Source: three-view drawing plus pictorial views. Frame: mm from the lowest corner of the part. Coordinates: 2 decimals unless noted, no trailing zeros. Loops run counter-clockwise (first coordinate to the right, second up) from the corner with the lowest first, then second, coordinate; pieces in that order, holes last. Notation, with made-up numbers: (75.25, 36) - (114.25, 36) arc R21 ccw to (114.25, 46) - close; hole circle Ø5 at (2, 70.5). An arc over 180 degrees is marked (long way). Return JSON: item names as keys, results as strings.
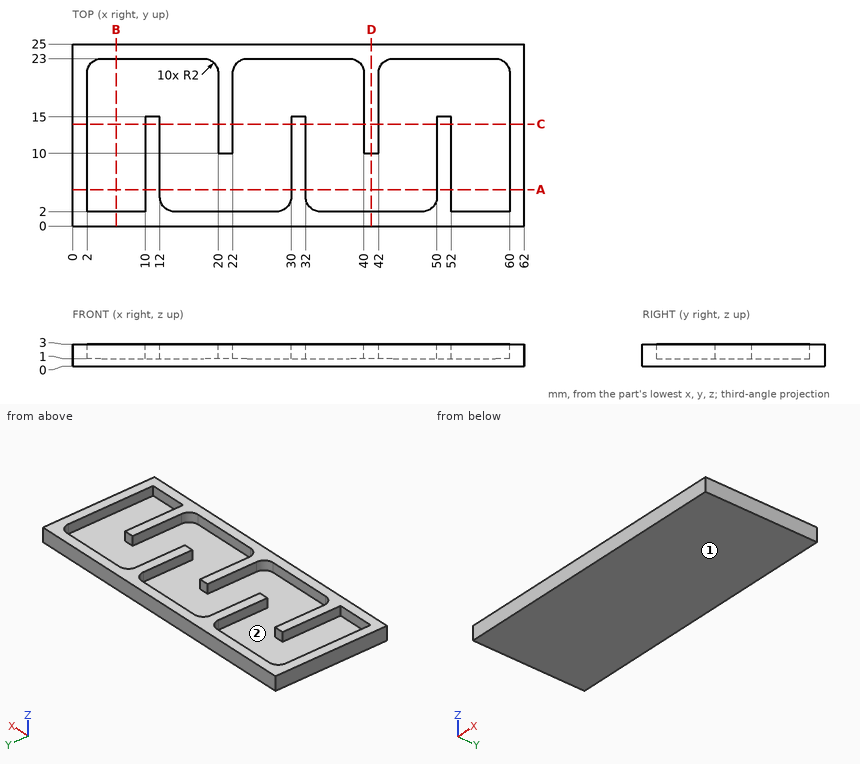
Item 1: Mould query, pull axis X, two halves, no side actions, for the marked faces 1 and 2. Classes: +X half, -X half, draft (parallel to the pull), parting line (faces both ways), or undercut.
Worked out:
{"face 1": "draft", "face 2": "undercut"}
Item 2: First-contact query: pin 1 Ø5 at (x, y) = (15, 20) entering from +Z. Flat tip, straight axial feed; report the tip coordinate or a pass-through.
Worked out:
{"pin 1": "z = 1"}
Item 3: Section query C-C, the plane y = 14. Return loops of the section in (x, z).
Worked out:
{"outline": "(0, 0) - (62, 0) - (62, 3) - (60, 3) - (60, 1) - (52, 1) - (52, 3) - (50, 3) - (50, 1) - (42, 1) - (42, 3) - (40, 3) - (40, 1) - (32, 1) - (32, 3) - (30, 3) - (30, 1) - (22, 1) - (22, 3) - (20, 3) - (20, 1) - (12, 1) - (12, 3) - (10, 3) - (10, 1) - (2, 1) - (2, 3) - (0, 3) - close"}
Item 4: Ray query, probe 1 along X at (y, z) = (9, 1.8); probe 2 along X at (y, z) = (16, 1.3); probe 3 along Y at (x, z) = (44, 1.25). Return the intervals inside material, ascending. Write a range as from..to.
Worked out:
{"probe 1": "0..2, 10..12, 30..32, 50..52, 60..62", "probe 2": "0..2, 20..22, 40..42, 60..62", "probe 3": "0..2, 23..25"}
Item 5: Section query A-A, the plane y = 5. Return loops of the section in (x, z).
Worked out:
{"outline": "(0, 0) - (62, 0) - (62, 3) - (60, 3) - (60, 1) - (52, 1) - (52, 3) - (50, 3) - (50, 1) - (32, 1) - (32, 3) - (30, 3) - (30, 1) - (12, 1) - (12, 3) - (10, 3) - (10, 1) - (2, 1) - (2, 3) - (0, 3) - close"}
Item 6: Section query D-D, the plane x = 41. Return loops of the section in (y, z), and give its area (3 significant figures).
Worked out:
{"outline": "(0, 0) - (25, 0) - (25, 3) - (10, 3) - (10, 1) - (2, 1) - (2, 3) - (0, 3) - close", "area": "59.0 mm^2"}
Item 7: Section query B-B, the plane x = 6. Return loops of the section in (y, z).
Worked out:
{"outline": "(0, 0) - (25, 0) - (25, 3) - (23, 3) - (23, 1) - (2, 1) - (2, 3) - (0, 3) - close"}
